from build123d import *

# Parameters (mm, degrees)
F0_W     = 76.2
F0_H     = 50.8
F0_R     = 12.7
F1_DEPTH = 12.7
F2_W     = 6.35
F2_H     = 50.8
F3_DEPTH = 2.54
F5_DEPTH = 50.801


with BuildPart() as f1:
    # F0 (on Top) → F1 (new body)
    with BuildSketch(Plane.XY):
        Rectangle(F0_W, F0_H)
        Circle(F0_R, mode=Mode.SUBTRACT)
    extrude(amount=F1_DEPTH)

    # F2 (on face) → F3 (cut)
    with BuildSketch(Plane.XY.offset(12.7)):
        with Locations((-32.385, 0)):
            Rectangle(F2_W, F2_H)
        with BuildLine():
            Line((6.35, 25.4), (-6.35, 25.4))
            Line((-6.35, 25.4), (-6.35, 10.9985226281))
            ThreePointArc((-6.35, 10.9985226281), (0, 12.7), (6.35, 10.9985226281))
            Line((6.35, 10.9985226281), (6.35, 25.4))
        make_face()
        with BuildLine():
            Line((-6.35, -10.9985226281), (-6.35, -25.4))
            Line((-6.35, -25.4), (6.35, -25.4))
            Line((6.35, -25.4), (6.35, -10.9985226281))
            ThreePointArc((6.35, -10.9985226281), (0, -12.7), (-6.35, -10.9985226281))
        make_face()
    extrude(amount=-F3_DEPTH, mode=Mode.SUBTRACT)

    # F4 (on face) → F5 (cut, through all)
    with BuildSketch(Plane.XZ.offset(25.4)):
        Polygon((31.75, 12.7), (19.05, 12.7), (16.1170606325, 7.62), (34.6829393675, 7.62), align=None)
    extrude(amount=-F5_DEPTH, mode=Mode.SUBTRACT)


solid = f1.part
Verification items for the finished model (mm, model axes). A direction names the side the tool comes from. Give positions to 0.01 mm unless a question says otherwise; leave off trailing zeros. Loops run counter-clockwise (first coordinate to the right, second up) from the corner with the lowest first, then second, coordinate; pieces in that order, holes last.
1. Tool access check on faces 1 (the flat face through (38.1, 0, 6)), 2 (the flat face through (-29.21, 0, 11)), 3 (the flat face through (17.604, -0.356, 10.196)). Record the directions out of +Z, -Z, +X, -X, +Y, -Y that give a thin tool (end or side, any length) a straight path to the whole face; none if there is none.
Derived:
face 1: +Z, -Z, +X, +Y, -Y
face 2: +Z, +Y, -Y
face 3: +Y, -Y
2. Cross-section at A-A on x = 0. Record the cut outline in (y, z).
Derived:
outline: (-25.4, 0) - (-12.7, 0) - (-12.7, 10.16) - (-25.4, 10.16) - close; (12.7, 0) - (25.4, 0) - (25.4, 10.16) - (12.7, 10.16) - close
3. Release check for a two-part mould opening along Y. For faces 4 (the flat face through (8, 12, 0)), 5 (the cylindrical face through (-1.653, 12.592, 6.261)), 6 (the flat face through (-1, -25.4, 6)), 7 (the flat face through (-1, 25.4, 6)) record: +Y half, -Y half, draft (parallel to the pull), parting line (faces both ways), or undercut.
Derived:
face 4: draft
face 5: undercut
face 6: -Y half
face 7: +Y half
4. Material ranges on probe 1 along Y at (x, z) = (0, 4.25); probe 2 along X at (y, z) = (0, 7.75); probe 3 along X at (y, z) = (-5.5, 10.5), recorded low to high.
Derived:
probe 1: y = -25.4 to -12.7, 12.7 to 25.4
probe 2: x = -38.1 to -12.7, 12.7 to 16.19, 34.61 to 38.1
probe 3: x = -38.1 to -35.56, -29.21 to -11.45, 11.45 to 17.78, 33.02 to 38.1
5. Cross-section at D-D on z = 11.75. Record the cut outline in (x, y), and give its area (3 significant figures).
Derived:
outline: (-38.1, -25.4) - (-35.56, -25.4) - (-35.56, 25.4) - (-38.1, 25.4) - close; (-29.21, -25.4) - (-6.35, -25.4) - (-6.35, -11) arc R12.7 cw to (-6.35, 11) - (-6.35, 25.4) - (-29.21, 25.4) - close; (6.35, -25.4) - (18.5, -25.4) - (18.5, 25.4) - (6.35, 25.4) - (6.35, 11) arc R12.7 cw to (6.35, -11) - close; (32.3, -25.4) - (38.1, -25.4) - (38.1, 25.4) - (32.3, 25.4) - close
area: 2,000 mm2
6. Cross-section at C-C on y = 0. Record the cut outline in (x, z).
Derived:
outline: (-38.1, 0) - (-12.7, 0) - (-12.7, 12.7) - (-29.21, 12.7) - (-29.21, 10.16) - (-35.56, 10.16) - (-35.56, 12.7) - (-38.1, 12.7) - close; (12.7, 0) - (38.1, 0) - (38.1, 12.7) - (31.75, 12.7) - (34.68, 7.62) - (16.12, 7.62) - (19.05, 12.7) - (12.7, 12.7) - close
7. Cross-section at B-B on z = 1. Record the cut outline in (x, y), and give its area (3 significant figures).
Derived:
outline: (-38.1, -25.4) - (38.1, -25.4) - (38.1, 25.4) - (-38.1, 25.4) - close; hole circle Ø25.4 at (0, 0)
area: 3,360 mm2
8. Go/stop test with a flat-tipped pin: P1, Ø6.5, axis at x = 1, y = -21, coming from the +Z side. Record where the tip stops, or that it passes through.
Derived:
P1: stops at z = 10.16
